Autodesk Inventor part; units mm, degrees
ref_plane "YZ Plane" through (0, 0, 0) normal (1, 0, 0) x (0, 1, 0)
ref_plane "XZ Plane" through (0, 0, 0) normal (0, 1, 0) x (-1, 0, 0)
ref_plane "XY Plane" through (0, 0, 0) normal (0, 0, 1) x (1, 0, 0)
sketch "スケッチ1" plane through (0, 0, 0) normal (0, 0, 1) x (1, 0, 0)
  circle A0 centre (0, 0) radius 1.5
  circle A1 centre (0, 0) radius 3.1
  line L0 (-0.4, 0) -> (0.4, 0)
  line L1 (0.4, 0) -> (0.4, -3.1)
  line L2 (0.4, -3.1) -> (-0.4, -3.1)
  line L3 (-0.4, -3.1) -> (-0.4, 0)
  line L4 (-1.0712, 1.05) -> (1.0712, 1.05)
  circle A2 centre (0, 0) radius 15
  circle A3 centre (0, 0) radius 13.4
  line L5 (-1.4605, 1.0815) -> (-1.1105, 1.4385)
  line L6 (-1.1105, 1.4385) -> (0.175, 0.1785)
  line L7 (0.175, 0.1785) -> (-0.175, -0.1785)
  line L8 (-0.175, -0.1785) -> (-1.4605, 1.0815)
  line L9 (1.4605, 1.0815) -> (1.1105, 1.4385)
  line L10 (1.1105, 1.4385) -> (-0.175, 0.1785)
  line L11 (-0.175, 0.1785) -> (0.175, -0.1785)
  line L12 (0.175, -0.1785) -> (1.4605, 1.0815)
  line L13 (0, 0) -> (-1.0712, 1.05) construction
  line L14 (1.0712, 1.05) -> (0, 0) construction
  point P0 (0.4, -1.4457)
  point P1 (0.4, -3.0741)
  point P2 (-0.4, -3.0741)
  point P3 (-0.4, -1.4457)
  point P4 (-0.7141, 1.05)
  point P5 (0.7141, 1.05)
  point P6 (1.2312, 0.8568)
  point P7 (-1.2312, 0.8568)
  dimension "SHAFT_D" = 3
  dimension "SLIT" = 0.8
  dimension "HUB_THIN" = 1.6
  dimension "d3" = 1.05
  dimension "WHEEL_D" = 30
  dimension "d5" = 1.6
  dimension "d18" = 0.5
  dimension "d19" = 1.8
extrude "ハブ＆リム" add sketch "スケッチ1" along normal blind 10 contours A0 L12 L9 L10 L6 L5 L8 L3 A1 L1 | L10 L4 L6 A0 | A2
sketch "スケッチ2" plane through (0, 0, 0) normal (0, 0, 1) x (1, 0, 0)
  line L0 (-0.8, 2.6) -> (0.8, 2.6)
  line L1 (0.8, 2.6) -> (0.8, 13.4)
  line L2 (0.8, 13.4) -> (-0.8, 13.4)
  line L3 (-0.8, 13.4) -> (-0.8, 2.6)
  circle A0 centre (0, 0) radius 13.4
  point P0 (0, 13.4)
  dimension "d8" = 1.6
  dimension "d9" = 2.6
extrude "スポーク" add sketch "スケッチ2" along normal up to surface (10 mm away) contours L3 A0 L1 L0 | L3 L2 A0 | A0 L2 L1 picked at (0, 6.2)
pattern_circular "円形状パターン1" count 3 over 360 about axis through (0, 0, -10) along (0, 0, 1) of "スポーク"
chamfer "面取り1" distance 0.3 angle 45 3 edges at (-1.4109, -0.5094, 10) (0, 1.05, 10) (1.4109, -0.5094, 10)
equation "\"d5\" = HUB_THIN"
properties part number "D-Shaft_Wheel1"
Input: part model. Units: mm. Frame: model coordinates. A direction names the side the tool comes from. Give positions to 0.01 mm unless a question says otherwise; leave off trailing zeros. Order: outer loops, then holes, each group sorted by start corner. A loop starts at its lowest first (then second) coordinate and runs counter-clockwise, first axis right, second up. Notation, with made-up numbers: M 51.5,-40 L 78.5,-40 A10 cw 78.5,-27 Z; hole C 65.25,-10 d7. An arc over 180 degrees is marked long. Return JSON: item names as keys, results as strings.
1) Access query for faces 4 (the face through (-1.53, -0.54, 9.82)), 5 (the face through (7.552, -3.436, 4.93)). Directions: +Z, -Z, +X, -X, +Y, -Y. A direction counts if a zero-diameter tool reaches every point of the face in a straight line with its end or side. Return the directions, or none.
Taken from the geometry:
{"face 4": "+Z", "face 5": "+Z, -Z"}
2) Section query B-B on z = 1. Count the separate pieces of the cut face and the enclosed holes in it, and give its area (3 significant figures).
Taken from the geometry:
{"separate pieces": "1", "enclosed holes": "3", "area": "214 mm2"}
3) Contact query for flat-ended pins moving along their axis: pin 1 (3 mm diameter, centred on y = 9, z = 3.5, fed in from -X); pin 2 (6 mm diameter, centred on y = 9.5, z = 5.5, fed in from +X); pin 3 (1.8 mm diameter, centred on y = -2.5, z = 6, fed in from -X). Output: stop coordinate, or through.
Taken from the geometry:
{"pin 1": "stops at x = -12.99", "pin 2": "stops at x = 13.52", "pin 3": "stops at x = -14.91"}
4) Section query A-A on x = 0. Output: boundary loops of the cut face in (y, z), and give its area (3 significant figures).
Taken from the geometry:
{"outline": "M -15,0 L -13.4,0 L -13.4,10 L -15,10 Z; M 1.05,0 L 15,0 L 15,10 L 1.35,10 L 1.05,9.7 Z", "area": "155 mm2"}
5) Section query D-D on y = -9.75. Output: boundary loops of the cut face in (x, z).
Taken from the geometry:
{"outline": "M -11.4,0 L -9.19,0 L -9.19,10 L -11.4,10 Z; M 9.19,0 L 11.4,0 L 11.4,10 L 9.19,10 Z"}
6) Mould query, pull axis X, two halves, no side actions, for faces 1 (the face through (-7.426, -3.364, 4.93)), 2 (the face through (-2, 0, 10)), 3 (the face through (-14.985, -0.66, 4.93)). Classes: released by +X, released by -X, zero draft, split by the parting line, or undercut.
Taken from the geometry:
{"face 1": "undercut", "face 2": "zero draft", "face 3": "split by the parting line"}
7) Section query C-C on y = 2.25. Output: boundary loops of the cut face in (x, z), and give its area (3 significant figures).
Taken from the geometry:
{"outline": "M -14.83,0 L -13.21,0 L -13.21,10 L -14.83,10 Z; M -2.13,0 L 2.13,0 L 2.13,10 L -2.13,10 Z; M 13.21,0 L 14.83,0 L 14.83,10 L 13.21,10 Z", "area": "75.1 mm2"}
8) Line query: L1, parallel to X at y = 10, z = 4.5; L2, parallel to Y at x = 8, z = 9.25; L3, parallel to Y at x = 4, z = 5.5. Output: solid intervals per line, ascending. Write a range as [from, to].
Taken from the geometry:
{"L1": "x = [-11.18, -8.92], [-0.8, 0.8], [8.92, 11.18]", "L2": "y = [-12.69, -10.75], [-5.54, -3.7], [10.75, 12.69]", "L3": "y = [-14.46, -12.79], [-3.23, -1.39], [12.79, 14.46]"}
